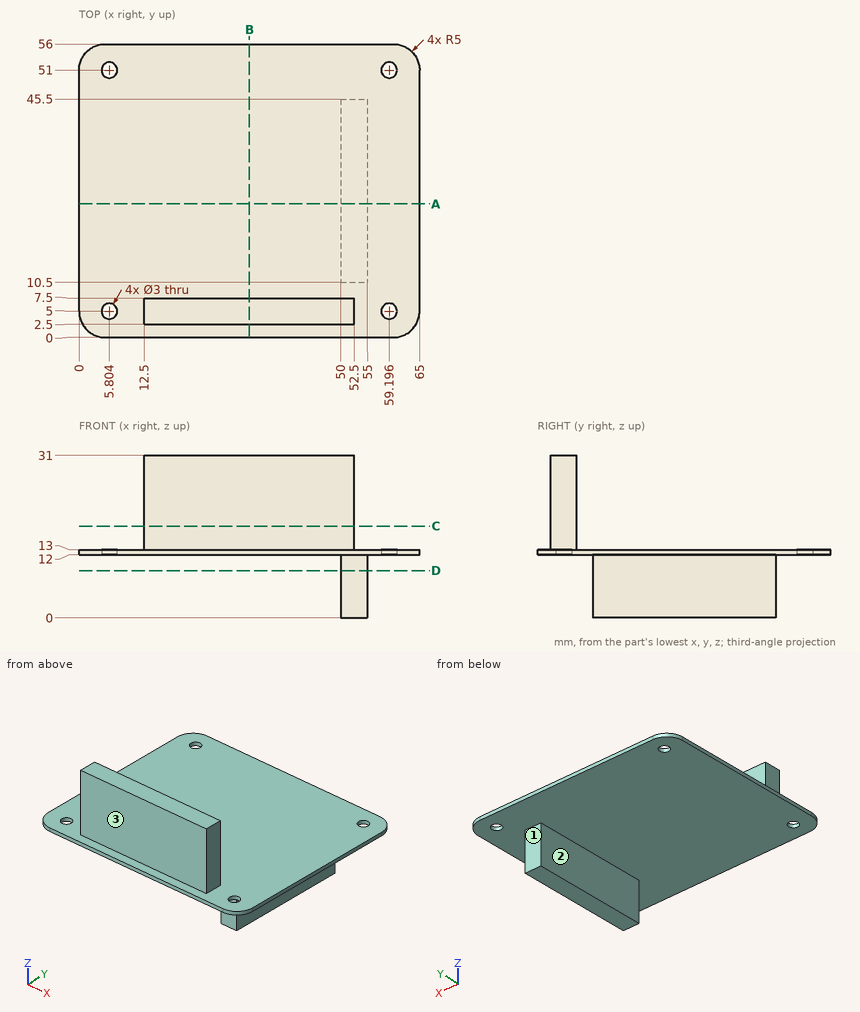
The drawing under review shows one solid part. Ordinate dimensions are in mm from its lowest x, y, z. A direction names the side the tool comes from. Coordinates: 2 decimals unless noted, no trailing zeros. Write each loop counter-clockwise with the first axis right and the second up, starting at its lowest first coordinate (ties: lowest second). Pieces come first, ordered by that corner, then holes. Notation, with made-up numbers: M 57,44.25 L 75,44.25 A15 ccw 75,64.25 Z; hole C -30.5,31 d11. An arc over 180 degrees is marked long. Answer as a JSON object with one key per item and string values.
Item 1: Add section C-C, the plane z = 17.5. Give the boundary of the cut face in (x, y), and give its area (3 significant figures).
Outcome:
{"outline": "M 12.5,2.5 L 52.5,2.5 L 52.5,7.5 L 12.5,7.5 Z", "area": "200 mm²"}
Item 2: Machinability: for the marked faces 1, 2 and 3, which of the approach directions +Z, -Z, +X, -X, +Y, -Y give a long, thin tool a straight path to every point of the face, cutting with its end or side? Answer none if there is none.
Outcome:
{"face 1": "-Z, +X, -X, +Y", "face 2": "-Z, -X, +Y, -Y", "face 3": "+Z, +X, -X, -Y"}
Item 3: Add section A-A, the plane y = 25.5. Give the boundary of the cut face in (x, z).
Outcome:
{"outline": "M 0,12 L 50,12 L 50,0 L 55,0 L 55,12 L 65,12 L 65,13 L 0,13 Z"}
Item 4: Add section B-B, the plane x = 32.5. Give the boundary of the cut face in (y, z).
Outcome:
{"outline": "M 0,12 L 56,12 L 56,13 L 7.5,13 L 7.5,31 L 2.5,31 L 2.5,13 L 0,13 Z"}
Item 5: Add section D-D, the plane z = 9. Give the boundary of the cut face in (x, y), and give its area (3 significant figures).
Outcome:
{"outline": "M 50,10.5 L 55,10.5 L 55,45.5 L 50,45.5 Z", "area": "175 mm²"}
Item 6: Insertion check: pin 1 Ø17 at (x, y) = (34, 21.5) entering from -Z; pin 2 Ø1.5 at (y, z) = (4, 19.5) entering from -X; pin 3 Ø2.5 at (x, z) = (52.5, 8.5) entering from -Y. Each pin has a flat end and moves straight along its axis. Give the tip position at first contact, or say it passes through.
Outcome:
{"pin 1": "z = 12", "pin 2": "x = 12.5", "pin 3": "y = 10.5"}
Item 7: Wall thickness on probe 1 along Z at (x, y) = (27.5, 34); probe 2 along Y at (x, z) = (33, 22); probe 3 along X at (y, z) = (37, 11): over which ranges is each line inside the solid? List them lowest first.
Outcome:
{"probe 1": "12 to 13", "probe 2": "2.5 to 7.5", "probe 3": "50 to 55"}
